The model under review builds one solid part; all positions refer to its coordinate system, in mm. Face numbers are marked on the shaded views. A direction names the side the tool comes from. Coordinates: 2 decimals unless noted, no trailing zeros. Order: outer loops, then holes, each group sorted by start corner. A loop starts at its lowest first (then second) coordinate and runs counter-clockwise, first axis right, second up. Notation, with made-up numbers: (54, 27) - (73, 27) arc R19 cw to (73, 33) - close; hole circle Ø2 at (83.25, 36.25). An arc over 180 degrees is marked (long way). Answer in a Markdown table with one row per item.
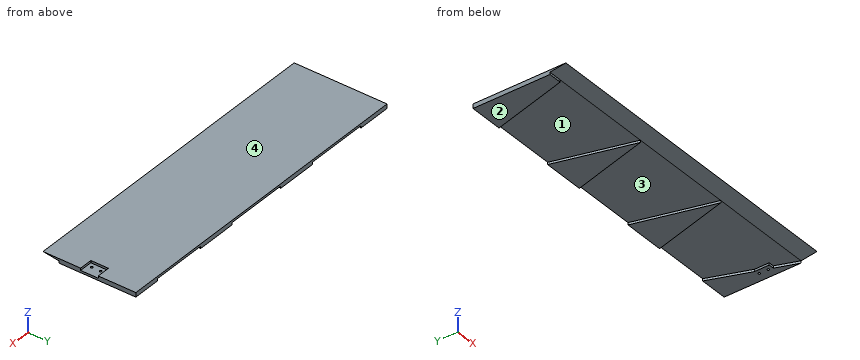
Autodesk Inventor part; units mm, degrees
ref_plane "YZ Plane" through (0, 0, 0) normal (1, 0, 0) x (0, 1, 0)
ref_plane "XZ Plane" through (0, 0, 0) normal (0, 1, 0) x (-1, 0, 0)
ref_plane "XY Plane" through (0, 0, 0) normal (0, 0, 1) x (1, 0, 0)
sketch "Sketch1" plane through (0, 0, 0) normal (0, 0, 1) x (1, 0, 0)
  line L0 (-37.1429, 20.9244) -> (432.7571, 20.9244)
  line L1 (432.7571, 20.9244) -> (432.7571, -112.4256)
  line L2 (432.7571, -112.4256) -> (-37.1429, -112.4256)
  line L3 (-37.1429, -112.4256) -> (-37.1429, 20.9244)
  point P0 (0, 0)
  dimension "d0" = 469.9
  dimension "d1" = 133.35
extrude "Extrusion1" add sketch "Sketch1" along normal blind 3.175
sketch "Sketch2" plane through (432.7571, -112.4256, 0) normal (1, 0, 0) x (0, 0, -1)
  line L0 (0, 133.35) -> (0, 0)
  line L1 (-3.175, 133.35) -> (0, 107.95)
  line L2 (-3.175, 0) -> (0, 22.86)
  line L3 (-3.175, 0) -> (0, 0)
  line L4 (0, 22.86) -> (0, 0)
  point P0 (0, 112.4256)
  dimension "d4" = 25.4
  dimension "d5" = 22.86
extrude "Extrusion3" cut sketch "Sketch2" against normal blind 476.25
sketch "Sketch4" plane through (0, 0, 0) normal (0, 0, -1) x (-1, 0, 0)
  line L0 (-432.7571, -89.5656) -> (37.1429, -89.5656)
  line L1 (37.1429, 20.9244) -> (-432.7571, 20.9244)
  line L2 (-432.7571, 20.9244) -> (-432.7571, -89.5656)
  line L3 (-432.7571, -89.5656) -> (37.1429, -89.5656)
  line L4 (37.1429, -89.5656) -> (37.1429, 20.9244)
  line L5 (37.1429, 20.9244) -> (-432.7571, 20.9244)
  line L6 (-432.7571, 20.9244) -> (-432.7571, -89.5656)
  line L7 (-282.4653, -89.5656) -> (-282.4653, 20.9244)
  line L8 (-132.1735, -89.5656) -> (-132.1735, 20.9244)
  line L9 (18.1183, -89.5656) -> (18.1183, 20.9244)
  line L10 (-282.4653, -89.5656) -> (-312.071, 20.9244)
  line L11 (-432.7571, -89.5656) -> (-392.5421, 20.9244)
  line L12 (-282.4653, -89.5656) -> (-252.8596, 20.9244)
  line L13 (-132.1735, -89.5656) -> (-161.7792, 20.9244)
  line L14 (-132.1735, -89.5656) -> (-102.5678, 20.9244)
  line L15 (18.1183, -89.5656) -> (-11.4874, 20.9244)
  line L16 (18.1183, 20.9244) -> (37.1429, 20.9244)
  line L17 (37.1429, 20.9244) -> (37.1429, -89.5656)
  line L18 (37.1429, -89.5656) -> (18.1183, -89.5656)
  line L19 (18.1183, -89.5656) -> (18.1183, 20.9244)
  point P0 (0, 0)
  dimension "d10" = 150.2918
  dimension "d11" = 150.2918
  dimension "d12" = 150.2918
  dimension "d13" = 20
  dimension "d14" = 15
  dimension "d15" = 15
extrude "Extrusion4" add sketch "Sketch4" along normal blind 3.175 contours L2 L1 L11 | L10 L1 L7 | L7 L1 L12 | L13 L1 L8 | L8 L1 L14 | L15 L1 L9
sketch "Sketch5" plane through (0, 0, 0) normal (0, 0, -1) x (-1, 0, 0)
  line L0 (18.1183, 20.9244) -> (18.1183, -89.5656)
  line L1 (18.1183, -89.5656) -> (37.1429, -89.5656)
  line L2 (37.1429, -89.5656) -> (37.1429, 20.9244)
  line L3 (37.1429, 20.9244) -> (18.1183, 20.9244)
  line L4 (18.1183, 20.9244) -> (37.1429, 20.9244)
  line L5 (37.1429, 20.9244) -> (37.1429, -89.5656)
  line L6 (37.1429, -89.5656) -> (18.1183, -89.5656)
  line L7 (18.1183, -89.5656) -> (18.1183, 20.9244)
  point P0 (0, 0)
sketch "Sketch6" plane through (0, 0, 3.175) normal (0, 0, 1) x (1, 0, 0)
  line L0 (-37.1429, 20.9244) -> (-18.1183, 20.9244)
  line L1 (-18.1183, 20.9244) -> (-18.1183, -89.5656)
  line L2 (-18.1183, -89.5656) -> (-37.1429, -89.5656)
  line L3 (-37.1429, -89.5656) -> (-37.1429, 20.9244)
  point P0 (0, 0)
  dimension "d18" = 110.49
  dimension "d19" = 19.0246
extrude "Extrusion5" add sketch "Sketch6" against normal blind 6.35
sketch "Sketch9" plane through (0, 0, 3.175) normal (0, 0, 1) x (1, 0, 0)
  line L0 (432.7571, 20.9244) -> (432.7571, -112.4256)
  line L1 (432.7571, -33.0506) -> (413.7071, -33.0506)
  line L2 (413.7071, -33.0506) -> (413.7071, -58.4506)
  line L3 (413.7071, -58.4506) -> (432.7571, -58.4506)
  line L4 (432.7571, -58.4506) -> (432.7571, -33.0506)
  point P0 (0, 0)
  dimension "d38" = 25.4
  dimension "d39" = 19.05
  dimension "d40" = 53.975
extrude "Extrusion8" cut sketch "Sketch9" against normal blind 3.175
sketch "Sketch10" plane through (0, 0, 0) normal (0, 0, 1) x (1, 0, 0)
  line L0 (413.7071, -37.2262) -> (421.4322, -58.4506)
  line L1 (432.7571, -33.0506) -> (413.7071, -33.0506)
  line L2 (413.7071, -33.0506) -> (413.7071, -37.2262)
  line L3 (413.7071, -37.2262) -> (421.4322, -58.4506)
  line L4 (413.7071, -58.4506) -> (413.7071, -37.2262)
  line L5 (421.4322, -58.4506) -> (413.7071, -58.4506)
  circle A0 centre (420.0571, -39.4006) radius 1.5875
  circle A1 centre (420.0571, -52.1006) radius 1.5875
  point P0 (0, 0)
  dimension "d43" = 12.7
  dimension "d44" = 6.35
  dimension "d45" = 3.175
  dimension "d46" = 3.175
  dimension "d47" = 6.35
extrude "Extrusion9" add sketch "Sketch10" against normal blind 3.175 contours L0 A1 L5 L4 | L0 A1 picked at (419.0163, -52.1007)
extrude "Extrusion10" cut sketch "Sketch10" against normal blind 3.175 contours A1 L0 | L0 A1 | A0
properties part number "bottom panel left"
Item 1: We need section A-A, the plane z = -1.5. Write out the cut boundary in (x, y) (1 decimal), then the cut area to 3 significant figures.
Check values:
| item | result |
|---|---|
| outline | (-37.1, -89.6) - (-18.1, -89.6) - (11.5, 20.9) - (-37.1, 20.9) - close; (102.6, 20.9) - (132.2, -89.6) - (161.8, 20.9) - close; (252.9, 20.9) - (282.5, -89.6) - (312.1, 20.9) - close; (392.5, 20.9) - (413.7, -37.2) - (413.7, -58.5) - (421.4, -58.5) - (432.8, -89.6) - (432.8, 20.9) - close; hole circle Ø3.2 at (420.1, -52.1); hole circle Ø3.2 at (420.1, -39.4) |
| area | 12,600 mm^2 |
Item 2: We need section C-C, the plane x = 339. Write out the cut boundary in (y, z) (3 decimals).
Check values:
| item | result |
|---|---|
| outline | (-112.426, 3.175) - (-89.566, 0) - (20.924, 0) - (20.924, 3.175) - close |
Item 3: We need section D-D, the plane y = -19.5. Write out the cut boundary in (x, z) (3 decimals).
Check values:
| item | result |
|---|---|
| outline | (-37.143, -3.175) - (0.656, -3.175) - (0.656, 0) - (113.399, 0) - (113.399, -3.175) - (150.948, -3.175) - (150.948, 0) - (263.691, 0) - (263.691, -3.175) - (301.239, -3.175) - (301.239, 0) - (407.255, 0) - (407.255, -3.175) - (432.757, -3.175) - (432.757, 3.175) - (-37.143, 3.175) - close |
Item 4: To check wall thickness, follow line 1 (X direction, y = -18.5, z = -2.5); line 2 (X direction, y = -62, z = -2.25); line 3 (Z direction, x = 172, y = 15) (3 decimals). State the ranges of each line that lie inside material, in increasing order. Write a range as from..to.
Check values:
| item | result |
|---|---|
| line 1 | -37.14..0.92, 113.13..151.22, 263.42..301.51, 406.89..432.76 |
| line 2 | -37.14..-10.73, 124.79..139.56, 275.08..289.85, 422.72..432.76 |
| line 3 | 0..3.175 |
Item 5: Mouldability with a two-part tool opening along X and no side actions: class the marked faces 1 and 2 as +X half, -X half, draft (parallel to the pull), parting line (faces both ways), or undercut.
Check values:
| item | result |
|---|---|
| face 1 | undercut |
| face 2 | draft |
Item 6: Clearance check with flat-ended pins moving along their axes: pin 1 Ø2.5 at (x, y) = (420.06, -39.4) entering from -Z (3 decimals); pin 2 Ø2.5 at (x, z) = (418, -2.5) entering from -Y; pin 3 Ø2.5 at (y, z) = (-48, 1.5) entering from +X; pin 4 Ø1.6 at (x, z) = (-27.5, -1.5) entering from -Y. State where each tip first meets the part, or that it passes through.
Check values:
| item | result |
|---|---|
| pin 1 | through |
| pin 2 | y = -58.45 |
| pin 3 | x = 413.71 |
| pin 4 | y = -89.57 |
Item 7: Tool access review of the marked faces 3 and 4: name each direction out of +Z, -Z, +X, -X, +Y, -Y from which nothing blocks a thin tool from reaching the whole face with its end or side.
Check values:
| item | result |
|---|---|
| face 3 | -Z, -Y |
| face 4 | +Z, +X, -X, +Y, -Y |
